Autodesk Inventor part; units mm, degrees
ref_plane "YZ Plane" through (0, 0, 0) normal (1, 0, 0) x (0, 1, 0)
ref_plane "XZ Plane" through (0, 0, 0) normal (0, 1, 0) x (-1, 0, 0)
ref_plane "XY Plane" through (0, 0, 0) normal (0, 0, 1) x (1, 0, 0)
sketch "Sketch1" plane through (0, 0, 0) normal (0, 0, 1) x (1, 0, 0)
  line L0 (-11.999, -0.0009) -> (209.001, -0.0009) construction
  circle A0 centre (47.001, -0.0009) radius 42.5 construction
  circle A1 centre (132.001, -0.0009) radius 42.5 construction
  circle A2 centre (47.001, -0.0009) radius 47.5625 construction
  circle A3 centre (132.001, -0.0009) radius 47.5625 construction
  arc A4 (82.1177, 32.0773) -> (-0.5615, -0.0019) centre (47.001, -0.0009) ccw
  arc A5 (179.5635, -0.0009) -> (96.8843, 32.0773) centre (132.001, -0.0009) ccw
  arc A6 (-0.5615, -0.0019) -> (82.1177, -32.079) centre (47.001, -0.0009) ccw
  arc A7 (96.8843, -32.079) -> (179.5635, -0.0009) centre (132.001, -0.0009) ccw
  arc A8 (75.7238, 47.5616) -> (-8.5615, -0.0015) centre (47.001, -0.0009) ccw
  arc A9 (187.5635, -0.0009) -> (103.2782, 47.5616) centre (132.001, -0.0009) ccw
  line L1 (47.001, 47.5616) -> (132.001, 47.5616) construction
  arc A10 (75.7238, 47.5616) -> (103.2782, 47.5616) centre (89.501, 70.3754) ccw
  arc A11 (-8.5615, -0.0015) -> (75.7238, -47.5634) centre (47.001, -0.0009) ccw
  arc A12 (103.2782, -47.5634) -> (187.5635, -0.0009) centre (132.001, -0.0009) ccw
  arc A13 (103.2782, -47.5634) -> (75.7238, -47.5634) centre (89.501, -70.3772) ccw
  arc A14 (82.1177, 32.0773) -> (96.8843, 32.0773) centre (89.501, 38.8217) ccw
  line L2 (82.1177, 32.0773) -> (96.8843, 32.0773) construction
  arc A15 (96.8843, -32.079) -> (82.1177, -32.079) centre (89.501, -38.8234) ccw
  point P0 (89.501, 21.3519)
  point P1 (46.9513, 55.5616)
  point P2 (132.0501, 55.5616)
  dimension "d5" = 221
  dimension "d6" = 85
  dimension "d7" = 85
  dimension "d8" = 85
  dimension "d9" = 95.125
  dimension "d10" = 95.125
  dimension "d12" = 8
  dimension "d20" = 10
extrude "Extrusion1" add sketch "Sketch1" along normal blind 50
sketch "Sketch2" plane through (0, 0, 50) normal (0, 0, 1) x (1, 0, 0)
  arc A0 (75.7238, 47.5616) -> (75.7238, -47.5634) centre (47.001, -0.0009) ccw
  arc A1 (75.7238, 47.5616) -> (103.2782, 47.5616) centre (89.501, 70.3754) ccw
  arc A2 (103.2782, -47.5634) -> (103.2782, 47.5616) centre (132.001, -0.0009) ccw
  arc A3 (103.2782, -47.5634) -> (75.7238, -47.5634) centre (89.501, -70.3772) ccw
  point P0 (0, 0)
extrude "Extrusion2" add sketch "Sketch2" along normal blind 8
fillet "Fillet1" radius 5 4 edges at (89.501, -43.7261, 58) (187.5635, -0.0009, 58) (89.501, 43.7243, 58) (-8.5615, -0.0009, 58)
sketch "Sketch3" plane through (0, 0, 0) normal (0, 0, -1) x (-1, 0, 0)
  line L0 (8.5615, -0.0009) -> (-187.5635, -0.0009) construction
  arc A0 (-103.2782, 47.5616) -> (-103.2782, -47.5634) centre (-132.001, -0.0009) ccw construction
  arc A1 (-75.7238, -47.5634) -> (-75.7238, 47.5616) centre (-47.001, -0.0009) ccw construction
  point P0 (0, 0)
  dimension "d27" = 196.125
equation "\"d7\" = d6"
equation "\"d8\" = d6"
equation "\"d10\" = d9"
properties part number "Gehaeuse_V2"
CAD build for the part. Positions are in the model's coordinates, mm. A direction names the side the tool comes from. Give positions to 0.01 mm unless a question says otherwise; leave off trailing zeros. Order: outer loops, then holes, each group sorted by start corner. A loop starts at its lowest first (then second) coordinate and runs counter-clockwise, first axis right, second up. Notation, with made-up numbers: (-34, -30.5) -> (-22, -30.5) arc R27 ccw to (-22, 6.5) -> close; hole circle Ø2 at (-19.75, 49). An arc over 180 degrees is marked (long way). Return JSON: item names as keys, results as strings.
Q1. Saw through at A-A (z = 9.5). Write the cut outline in (x, y) (1 decimal), then the cut area to 3 significant figures.
Working result:
{"outline": "(-8.6, 0) arc R55.6 ccw to (75.7, -47.6) arc R26.7 cw to (103.3, -47.6) arc R55.6 ccw to (187.6, 0) arc R55.6 ccw to (103.3, 47.6) arc R26.7 cw to (75.7, 47.6) arc R55.6 ccw to start; hole (-0.6, 0) arc R47.6 ccw to (82.1, -32.1) arc R10 cw to (96.9, -32.1) arc R47.6 ccw to (179.6, 0) arc R47.6 ccw to (96.9, 32.1) arc R10 cw to (82.1, 32.1) arc R47.6 ccw to start", "area": "4,260 mm²"}
Q2. Flat gauge pins, fed straight in: pin 1 (10 mm diameter, centred on y = -40, z = 10.5, fed in from -X); pin 2 (5 mm diameter, centred on x = 160, y = 27, fed in from -Z); pin 3 (6 mm diameter, centred on y = -25.5, z = 10, fed in from -X). Where does each tip first touch, or does it go through?
Working result:
{"pin 1": "x = 3.85", "pin 2": "z = 50", "pin 3": "x = -3.8"}
Q3. Drill centre lines: line 1 (X direction, y = 40, z = 18); line 2 (X direction, y = -39, z = 20); line 3 (Z direction, x = 61, y = -21.5). Where is each one in solid material? Low to high.
Working result:
{"line 1": "8.44 to 21.27, 72.73 to 106.27, 157.73 to 170.56", "line 2": "7.42 to 19.77, 74.23 to 104.77, 159.23 to 171.58", "line 3": "50 to 58"}
Q4. Mould opens along Y. For faces 3 (the face through (89.298, -43.727, 26.129)), 4 (the face through (88, 1, 58)), 5 (the face through (89.704, 43.725, 26.129)), 6 (the face through (89.617, 28.822, 24.65)) say: pulls with the +Y half, pulls with the -Y half, needs draft (parallel to the pull), parting line crosses it, or undercut.
Working result:
{"face 3": "pulls with the -Y half", "face 4": "needs draft", "face 5": "pulls with the +Y half", "face 6": "undercut"}
Q5. Which spindle directions (+Z, -Z, +X, -X, +Y, -Y) get a long thin tool onto all of the face, cutting with end or side? Do faces 1 (the face through (88, 1, 50)), 2 (the face through (89, 29, 0)). Say none if no direction does.
Working result:
{"face 1": "-Z", "face 2": "-Z, +X, -X, +Y, -Y"}
